from build123d import *

# Parameters (mm, degrees)
EXTRUDE_1_DEPTH = 0.3
FILLET_1_R      = 0.5


with BuildPart() as part:
    # 草图1 → 凸台-拉伸1 (new body)
    with BuildSketch(Plane.XY):
        with BuildLine():
            Line((0, 0), (0, 12.3))
            ThreePointArc((0, 12.3), (0.205025253, 12.794974747), (0.7, 13))
            Line((0.7, 13), (2.94, 13))
            ThreePointArc((2.94, 13), (3.434974747, 12.794974747), (3.64, 12.3))
            Line((3.64, 12.3), (3.64, 0))
            Line((3.64, 0), (2.32, 0))
            Line((2.32, 0), (2.32, 7.16))
            ThreePointArc((2.32, 7.16), (1.82, 7.66), (1.32, 7.16))
            Line((1.32, 7.16), (1.32, 0))
            Line((1.32, 0), (0, 0))
        make_face()
    extrude(amount=EXTRUDE_1_DEPTH)

    # 圆角1
    # the kernel refuses this fillet: 0.5 mm, written as the material it takes off along each edge
    with BuildSketch(Plane(origin=(2.465643924, 0, 0.3), x_dir=(0, 0, -1), z_dir=(-1, 0, 0)), Plane(origin=(4.785643924, 0, 0.3), x_dir=(0, 0, -1), z_dir=(-1, 0, 0))) as fillet_1_piece_1:
        with BuildLine():
            CenterArc((0.5, -0.458257569), FILLET_1_R, 113.578178478, 66.421821522)
            Line((0, -0.458257569), (-0.01, -0.458257569))
            Line((-0.01, -0.458257569), (-0.01, 0))
            Line((-0.01, 0), (0, 0.01))
            ThreePointArc((0, 0.01), (0.15, 0.01), (0.296, 0.009165151))
            Line((0.296, 0.009165151), (0.3, 0))
        make_face()
    extrude(amount=3.611287847, mode=Mode.SUBTRACT)


solid = part.part
Model file for the job. Use its own axes, mm. Coordinates: 2 decimals unless noted, no trailing zeros. Loops run counter-clockwise (first coordinate to the right, second up) from the corner with the lowest first, then second, coordinate; pieces in that order, holes last. Notation, with made-up numbers: (-27.75, -8) -> (0.25, -8) arc R28 ccw to (0.25, 19) -> close; hole circle Ø5 at (-19, 19). An arc over 180 degrees is marked (long way). Use one line per item in the form item = value. Start each with the question number.
(1) Cut at C-C on x = 1.82. Give the cut face in (y, z), and give its area (3 significant figures).
(2) Cut at A-A on y = 1.25. Give the cut face in (x, z).
(3) Probe probe 1 along X at (y, z) = (5.5, 0.25); probe 2 along X at (y, z) = (7.5, 0.15); probe 3 along Y at (x, z) = (1.95, 0.2). List the from-to ranges inside material, lowest first. Write a range as from..to.
(4) Cut at B-B on z = 0.25. Give the cut face in (x, y), and give its area (3 significant figures).
Values:
q1.outline = (7.66, 0) -> (13, 0) -> (13, 0.3) -> (7.66, 0.3) -> close
q1.area = 1.60 mm2
q2.outline = (0, 0) -> (1.32, 0) -> (1.32, 0.3) -> (0, 0.3) -> close; (2.32, 0) -> (3.64, 0) -> (3.64, 0.3) -> (2.32, 0.3) -> close
q3.probe_1 = 0..1.32, 2.32..3.64
q3.probe_2 = 0..1.45, 2.19..3.64
q3.probe_3 = 7.64..13
q4.outline = (0, 0.24) -> (1.32, 0.24) -> (1.32, 7.16) arc R0.5 cw to (2.32, 7.16) -> (2.32, 0.24) -> (3.64, 0.24) -> (3.64, 12.3) arc R0.7 ccw to (2.94, 13) -> (0.7, 13) arc R0.7 ccw to (0, 12.3) -> close
q4.area = 38.9 mm2
